from build123d import *

# Parameters (mm, degrees)
SKETCH1_R           = 31
BOSS_EXTRUDE1_DEPTH = 310
SKETCH2_R           = 30
CUT_EXTRUDE1_DEPTH  = 300
CUT_EXTRUDE2_DEPTH  = 7.5


with BuildPart() as part:
    # Sketch1 → Boss-Extrude1 (new body)
    with BuildSketch(Plane(origin=(0, 0, 0), x_dir=(1, 0, 0), z_dir=(0, 1, 0))):
        with Locations(Location((0, 0, 0), (0, 0, 270))):
            Circle(SKETCH1_R)
    extrude(amount=BOSS_EXTRUDE1_DEPTH)

    # Sketch2 → Cut-Extrude1 (cut)
    with BuildSketch(Plane(origin=(0, 310, 0), x_dir=(1, 0, 0), z_dir=(0, 1, 0))):
        with Locations(Location((0, 0, 0), (0, 0, 270))):
            Circle(SKETCH2_R)
    extrude(amount=-CUT_EXTRUDE1_DEPTH, mode=Mode.SUBTRACT)

    # Sketch3 → Cut-Extrude2 (cut)
    with BuildSketch(Plane.XZ):
        with BuildLine():
            Line((-26.278555896, -5), (-30.594117082, -5))
            ThreePointArc((-30.594117082, -5), (-31, 0), (-30.594117082, 5))
            Line((-30.594117082, 5), (-26.278555896, 5))
            ThreePointArc((-26.278555896, 5), (-26.75, 0), (-26.278555896, -5))
        make_face()
        with BuildLine():
            Line((-5, -26.278555896), (-5, -30.594117082))
            ThreePointArc((-5, -30.594117082), (0, -31), (5, -30.594117082))
            Line((5, -30.594117082), (5, -26.278555896))
            ThreePointArc((5, -26.278555896), (0, -26.75), (-5, -26.278555896))
        make_face()
        with BuildLine():
            Line((-5, 26.278555896), (-5, 30.594117082))
            ThreePointArc((-5, 30.594117082), (0, 31), (5, 30.594117082))
            Line((5, 30.594117082), (5, 26.278555896))
            ThreePointArc((5, 26.278555896), (0, 26.75), (-5, 26.278555896))
        make_face()
        with BuildLine():
            Line((26.278555896, 5), (30.594117082, 5))
            ThreePointArc((30.594117082, 5), (31, 0), (30.594117082, -5))
            Line((30.594117082, -5), (26.278555896, -5))
            ThreePointArc((26.278555896, -5), (26.75, 0), (26.278555896, 5))
        make_face()
    extrude(amount=-CUT_EXTRUDE2_DEPTH, mode=Mode.SUBTRACT)


solid = part.part
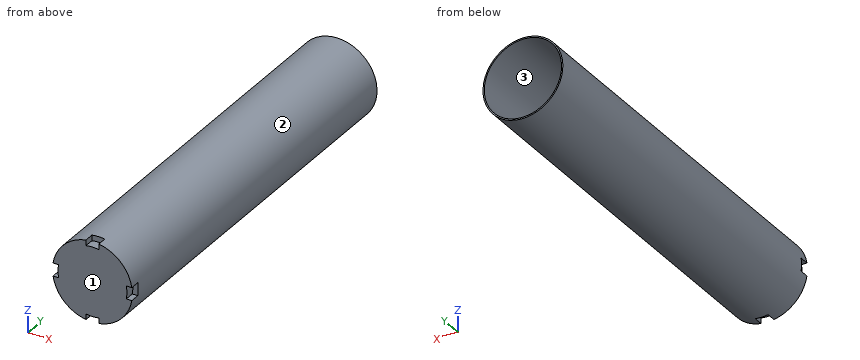
Source: CAD feature listing. Evaluate the final solid. Frame: model axes, mm. Face numbers are marked on the shaded views. Give positions to 0.01 mm unless a question says otherwise; leave off trailing zeros. Write each loop counter-clockwise with the first axis right and the second up, starting at its lowest first coordinate (ties: lowest second). Pieces come first, ordered by that corner, then holes. Notation, with made-up numbers: (89.5, 23.5) -> (143.5, 23.5) arc R6 ccw to (143.5, 34.5) -> close; hole circle Ø9 at (36.5, 87.5). An arc over 180 degrees is marked (long way). Return JSON: item names as keys, results as strings. Group by question number.
1. Section D-D, the plane x = -13.5. Output: boundary loops of the cut face in (y, z).
2. Section A-A, the plane x = 0. Output: boundary loops of the cut face in (y, z), then the cut area to 3 significant figures.
3. Material intervals for line 1 (X direction, y = 209, z = 0); line 2 (Y direction, x = -3, z = 17); line 3 (Z direction, x = -6, y = 142), sorted ascending. Write a range as from..to.
4. Mould query, pull axis X, two halves, no side actions, for the marked faces 1, 2 and 3. Classes: +X half, -X half, draft (parallel to the pull), parting line (faces both ways), or undercut.
5. Section C-C, the plane y = 193.5. Output: boundary loops of the cut face in (x, z), then the cut area to 3 significant figures.
6. Pin query (flat end, axial travel): pin 1 Ø1.3 at (y, z) = (3, 27.5) entering from +X; pin 2 Ø2.5 at (x, z) = (2.5, 29.5) entering from -Y; pin 3 Ø12 at (x, y) = (-19.5, 38) entering from +Z. Return the tip coordinate at first contact, or that it passes through.
7. Section B-B, the plane z = 0. Output: boundary loops of the cut face in (x, y), then the cut area to 3 significant figures.
Determined:
{
 "1": {"outline": "(0, -27.91) -> (310, -27.91) -> (310, -26.79) -> (10, -26.79) -> (10, 26.79) -> (310, 26.79) -> (310, 27.91) -> (0, 27.91) -> close"},
 "2": {"outline": "(0, -26.75) -> (7.5, -26.75) -> (7.5, -31) -> (310, -31) -> (310, -30) -> (10, -30) -> (10, 30) -> (310, 30) -> (310, 31) -> (7.5, 31) -> (7.5, 26.75) -> (0, 26.75) -> close", "area": "1,160 mm2"},
 "3": {"line 1": "x = -31..-30, 30..31", "line 2": "y = 0..10", "line 3": "z = -30.41..-29.39, 29.39..30.41"},
 "4": {"face 1": "draft", "face 2": "parting line", "face 3": "undercut"},
 "5": {"outline": "circle Ø62 at (0, 0); hole circle Ø60 at (0, 0)", "area": "192 mm2"},
 "6": {"pin 1": "stops at x = 15.49", "pin 2": "stops at y = 7.5", "pin 3": "stops at z = 27.91"},
 "7": {"outline": "(-31, 7.5) -> (-26.75, 7.5) -> (-26.75, 0) -> (26.75, 0) -> (26.75, 7.5) -> (31, 7.5) -> (31, 310) -> (30, 310) -> (30, 10) -> (-30, 10) -> (-30, 310) -> (-31, 310) -> close", "area": "1,160 mm2"}
}
